```python
from build123d import *

# Parameters (mm, degrees)
BOSS_EXTRUDE1_OUTLINE_R = 1.5
BOSS_EXTRUDE1_DEPTH     = 10
SKETCH3_R               = 3.25
CUT_EXTRUDE1_DEPTH      = 5
SKETCH4_R               = 3.25
CUT_EXTRUDE2_DEPTH      = 5


# Read off the part's stored shape, not the designer's step: Boss-Extrude1
with BuildPart() as part:
    # Boss-Extrude1 outline → Boss-Extrude1 (new body)
    with BuildSketch(Plane(origin=(0, 0, 0), x_dir=(1, 0, 0), z_dir=(0, 1, 0))):
        with BuildLine():
            ThreePointArc((-20, 18), (-25.525673356, 14.33814755), (-24.306613207, 7.822311322))
            Line((-24.306613207, 7.822311322), (-8.613226413, -8.355377356))
            ThreePointArc((-8.613226413, -8.355377356), (0, -12), (8.613226413, -8.355377356))
            Line((8.613226413, -8.355377356), (24.778677898, 8.371744559))
            ThreePointArc((24.778677898, 8.371744559), (25.374454979, 14.667439536), (20, 18))
            Line((20, 18), (-20, 18))
        make_face()
        Circle(BOSS_EXTRUDE1_OUTLINE_R, mode=Mode.SUBTRACT)
        with Locations((-20, 12)):
            Circle(BOSS_EXTRUDE1_OUTLINE_R, mode=Mode.SUBTRACT)
        with Locations((20, 12)):
            Circle(BOSS_EXTRUDE1_OUTLINE_R, mode=Mode.SUBTRACT)
    extrude(amount=BOSS_EXTRUDE1_DEPTH)

    # Sketch3 → Cut-Extrude1 (cut)
    with BuildSketch(Plane(origin=(0, 10, 0), x_dir=(1, 0, 0), z_dir=(0, 1, 0))):
        with Locations(Location((0, 0, 0), (0, 0, 270))):
            Circle(SKETCH3_R)
    extrude(amount=-CUT_EXTRUDE1_DEPTH, mode=Mode.SUBTRACT)

    # Sketch4 → Cut-Extrude2 (cut)
    with BuildSketch(Plane.XZ):
        with Locations(Location((20, -12, 0), (0, 0, 270))):
            Circle(SKETCH4_R)
        with Locations(Location((-20, -12, 0), (0, 0, 270))):
            Circle(SKETCH4_R)
    extrude(amount=-CUT_EXTRUDE2_DEPTH, mode=Mode.SUBTRACT)


solid = part.part
```
Geometry: final body of the model. Coordinates: model frame, mm. A direction names the side the tool comes from. Coordinates: 2 decimals unless noted, no trailing zeros. Order: outer loops, then holes, each group sorted by start corner. A loop starts at its lowest first (then second) coordinate and runs counter-clockwise, first axis right, second up. Notation, with made-up numbers: M 2,-38.75 L 40,-38.75 A20 cw 40,-28.75 Z; hole C 31,58.25 d5. An arc over 180 degrees is marked long. Answer in a Markdown table with one row per item. Add a question column.
Q1. Section query B-B on x = 0. Return the cut outline in (y, z).
Q2. Line query: L1, parallel to X at y = 6, z = -12; L2, parallel to X at y = 1.15, z = -12; L3, parallel to X at y = 3.75, z = 0. Output: solid intervals per line, ascending.
Q3. Mould query, pull axis X, two halves, no side actions, for faces 1 (the flat face through (19.3, 5, -10.5)), 2 (the cylindrical face through (-25.5, 4.9, -14.4)), 3 (the flat face through (16.58, 4.93, 0.11)). Classes: released by +X, released by -X, zero draft, split by the parting line, or undercut.
Q4. Section query C-C on z = -12. Return the cut outline in (x, y), and give its area (3 significant figures).
Q5. Contact query for flat-ended pins moving along their axis: P1, Ø1.5, axis at y = 5, z = 7, coming from the -X side; P2, Ø3.5, axis at x = -20, z = -12, coming from the -Y side; P3, Ø1.5, axis at y = 6, z = 3, coming from the -X side; P4, Ø2.5, axis at x = 20, z = -12, coming from the -Y side. Output: stop coordinate, or through.
Q6. Reachability of faces 4 (the flat face through (1.5, 5, 0.7)), 5 (the flat face through (-16.57, 4.93, 0.153)), 6 (the cylindrical face through (18.022, 2.465, -9.421)) from +Z, -Z, +X, -X, +Y, -Y: full face, straight path, thin tool, end or side. Return the list, or none.
Q7. Section query D-D on z = 0. Return the cut outline in (x, y), and give its area (3 significant figures).
Q8. Section query A-A on y = 4.25. Return the cut outline in (x, z).
Completed:
| question | item | result |
|---|---|---|
| 1 | outline | M 0,-18 L 10,-18 L 10,-3.25 L 5,-3.25 L 5,-1.5 L 0,-1.5 Z; M 0,1.5 L 5,1.5 L 5,3.25 L 10,3.25 L 10,12 L 0,12 Z |
| 2 | L1 | x = -26 to -21.5, -18.5 to 18.5, 21.5 to 26 |
| 2 | L2 | x = -26 to -23.25, -16.75 to 16.75, 23.25 to 26 |
| 2 | L3 | x = -16.72 to -1.5, 1.5 to 16.69 |
| 3 | face 1 | undercut |
| 3 | face 2 | released by -X |
| 3 | face 3 | released by +X |
| 4 | outline | M -26,0 L -23.25,0 L -23.25,5 L -21.5,5 L -21.5,10 L -26,10 Z; M -18.5,5 L -16.75,5 L -16.75,0 L 16.75,0 L 16.75,5 L 18.5,5 L 18.5,10 L -18.5,10 Z; M 21.5,5 L 23.25,5 L 23.25,0 L 26,0 L 26,10 L 21.5,10 Z |
| 4 | area | 425 mm2 |
| 5 | P1 | stops at x = -10.66 |
| 5 | P2 | stops at y = 5 |
| 5 | P3 | stops at x = -14.54 |
| 5 | P4 | passes through |
| 6 | face 4 | +Y |
| 6 | face 5 | +Z, -X, +Y, -Y |
| 6 | face 6 | -Y |
| 7 | outline | M -16.72,0 L -1.5,0 L -1.5,5 L -3.25,5 L -3.25,10 L -16.72,10 Z; M 1.5,0 L 16.69,0 L 16.69,10 L 3.25,10 L 3.25,5 L 1.5,5 Z |
| 7 | area | 287 mm2 |
| 8 | outline | M -24.31,-7.82 A6 ccw -20,-18 L 20,-18 A6 ccw 24.78,-8.37 L 8.61,8.36 A12 ccw -8.61,8.36 Z; hole C -20,-12 d6.5; hole C 0,0 d3; hole C 20,-12 d6.5 |
